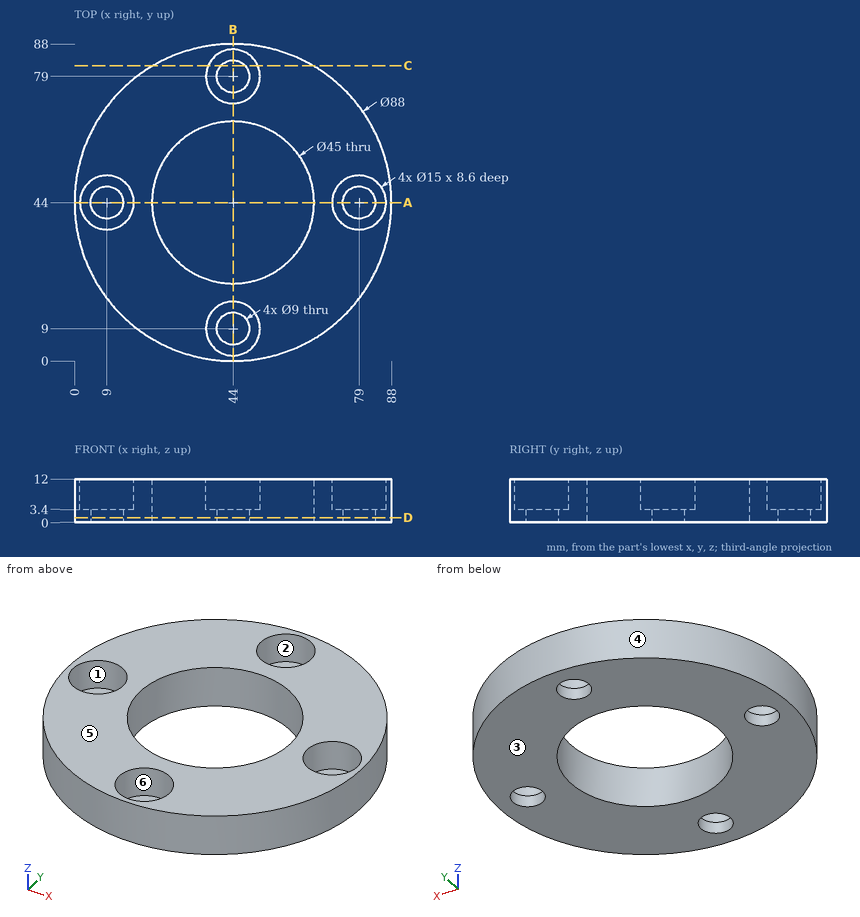
Source: three-view drawing plus pictorial views. Frame: mm from the lowest corner of the part. A direction names the side the tool comes from. Round coordinates to 2 decimals unless told otherwise and drop trailing zeros. Write each loop counter-clockwise with the first axis right and the second up, starting at its lowest first coordinate (ties: lowest second). Pieces come first, ordered by that corner, then holes. Notation, with made-up numbers: M 64,40.25 L 71,40.25 A25 ccw 71,71.25 Z; hole C 32.25,57 d9. An arc over 180 degrees is marked long. One line per item, written item: value. Start each with the question number.
Item 1: Section query D-D (z = 1.25). Return the cut outline in (x, y), plus the area to 3 significant figures.
Item 2: Section query A-A (y = 44). Return the cut outline in (x, z), plus the area to 3 significant figures.
Item 3: Ray query, L1, parallel to Y at x = 44, z = 8.5; L2, parallel to Y at x = 44, z = 1.9; L3, parallel to Y at x = 8, z = 8.5. Return the intervals inside material, ascending. Write a range as from..to.
Item 4: Set-up query: the marked faces 5 and 6. Return all of +Z, -Z, +X, -X, +Y, -Y with unobstructed straight access to the full face (end or side cutting, diameter ignored); none if empty.
Item 5: Pin query (flat end, axial travel): pin 1 (1.5 mm diameter, centred on x = 51.5, z = 6, fed in from -Y); pin 2 (4.5 mm diameter, centred on x = 41.5, y = 77, fed in from +Z); pin 3 (7 mm diameter, centred on x = 9, y = 44, fed in from -Z); pin 4 (6 mm diameter, centred on y = 28.5, z = 10, fed in from +X). Return the tip coordinate at first contact, or that it passes through.
Item 6: Mould query, pull axis Y, two halves, no side actions, for the marked faces 1, 2, 3 and 4. Classes: pulls with the +Y half, pulls with the -Y half, needs draft (parallel to the pull), parting line crosses it, or undercut.
Item 7: Section query C-C (y = 82). Return the cut outline in (x, z).
Result set:
1. outline: C 44,44 d88; hole C 9,44 d9; hole C 44,44 d45; hole C 44,9 d9; hole C 44,79 d9; hole C 79,44 d9
1. area: 4,240 mm²
2. outline: M 0,0 L 4.5,0 L 4.5,3.4 L 1.5,3.4 L 1.5,12 L 0,12 Z; M 13.5,0 L 21.5,0 L 21.5,12 L 16.5,12 L 16.5,3.4 L 13.5,3.4 Z; M 66.5,0 L 74.5,0 L 74.5,3.4 L 71.5,3.4 L 71.5,12 L 66.5,12 Z; M 83.5,0 L 88,0 L 88,12 L 86.5,12 L 86.5,3.4 L 83.5,3.4 Z
2. area: 197 mm²
3. L1: y = 0..1.5, 16.5..21.5, 66.5..71.5, 86.5..88
3. L2: y = 0..4.5, 13.5..21.5, 66.5..74.5, 83.5..88
3. L3: y = 18.7..36.57, 51.43..69.3
4. face 5: +Z, +X, -X, +Y, -Y
4. face 6: +Z
5. pin 1: stops at y = 0.52
5. pin 2: stops at z = 3.4
5. pin 3: passes through
5. pin 4: stops at x = 86.19
6. face 1: undercut
6. face 2: undercut
6. face 3: needs draft
6. face 4: parting line crosses it
7. outline: M 21.82,0 L 40.65,0 L 40.65,3.4 L 37.13,3.4 L 37.13,12 L 21.82,12 Z; M 47.35,0 L 66.18,0 L 66.18,12 L 50.87,12 L 50.87,3.4 L 47.35,3.4 Z
